Could you check a few things on this drawing? It's one solid part, dimensions in mm from its lowest x, y, z. A direction names the side the tool comes from. Give positions to 0.01 mm unless a question says otherwise; leave off trailing zeros. Order: outer loops, then holes, each group sorted by start corner. A loop starts at its lowest first (then second) coordinate and runs counter-clockwise, first axis right, second up.
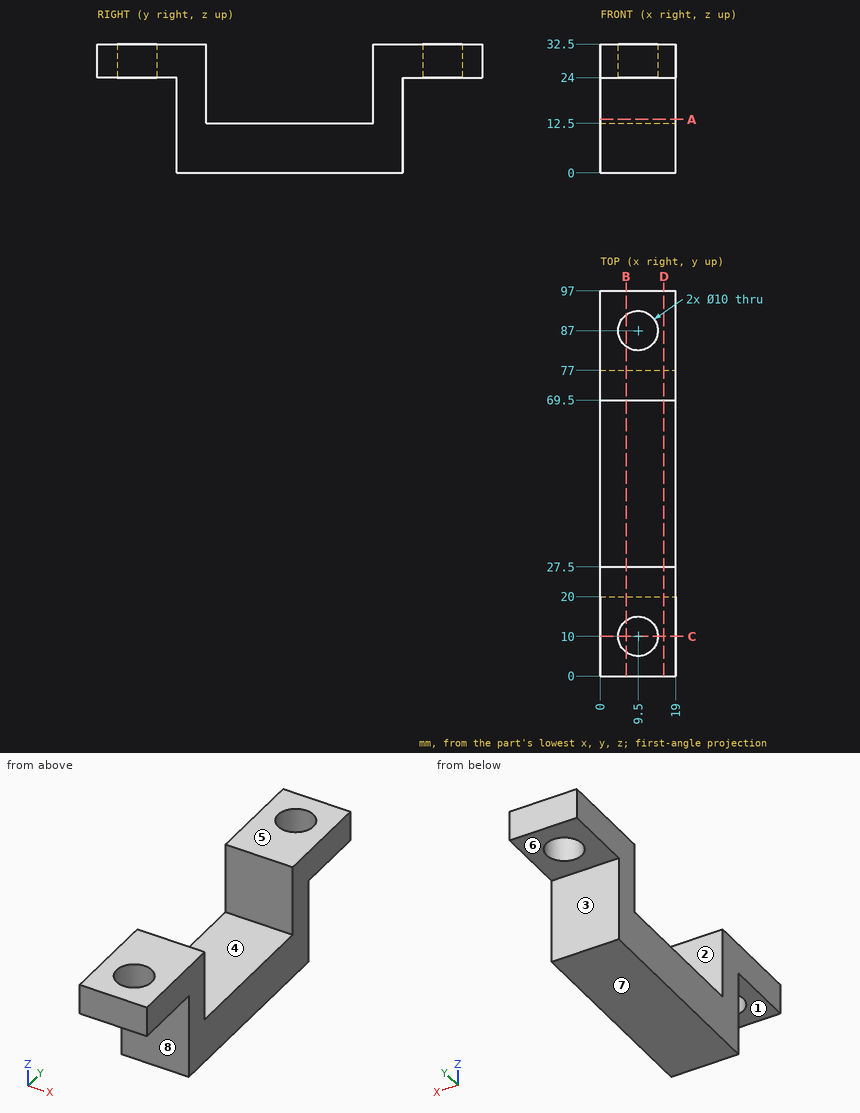
Q1. For the marked faces 4, 5, 6, 7 and 8, which set-ups out of +Z, -Z, +X, -X, +Y, -Y let a thin tool reach every point of the face, with its end or its side?
Filled sheet:
face 4: +Z, +X, -X
face 5: +Z, +X, -X, +Y, -Y
face 6: -Z, +X, -X, +Y
face 7: -Z, +X, -X, +Y, -Y
face 8: -Z, +X, -X, -Y
Q2. If we section it at A-A on z = 13.5: List the corners of the cut face in (x, y) for me.
Filled sheet:
outline: (0, 20) - (19, 20) - (19, 27.5) - (0, 27.5) - close; (0, 69.5) - (19, 69.5) - (19, 77) - (0, 77) - close
Q3. I'm going to push flat-ended pins straight in: P1, Ø9.5, axis at x = 5.5, z = 15, coming from the +Y side; P2, Ø9.5, axis at x = 13.5, y = 12, coming from the -Z side; P3, Ø9.5, axis at x = 12, z = 13, coming from the -Y side. Where does each tip first touch, or does it pass through?
Filled sheet:
P1: stops at y = 77
P2: stops at z = 24
P3: stops at y = 20
Q4. If we section it at C-C on y = 10: List the corners of the cut face in (x, z) for me.
Filled sheet:
outline: (0, 24) - (4.5, 24) - (4.5, 32.5) - (0, 32.5) - close; (14.5, 24) - (19, 24) - (19, 32.5) - (14.5, 32.5) - close
Q5. If we section it at D-D on x = 16: List the corners of the cut face in (y, z) for me.
Filled sheet:
outline: (0, 24) - (20, 24) - (20, 0) - (77, 0) - (77, 24) - (97, 24) - (97, 32.5) - (69.5, 32.5) - (69.5, 12.5) - (27.5, 12.5) - (27.5, 32.5) - (0, 32.5) - close
Q6. I need wall thicknesses on L1, parallel to Y at x = 9.5, z = 27.5; L2, parallel to Y at x = 13.5, z = 31; L3, parallel to Y at x = 2.75, z = 18. Which ranges of each line are inside material? Lowest first, please.
Filled sheet:
L1: y = 0 to 5, 15 to 27.5, 69.5 to 82, 92 to 97
L2: y = 0 to 7, 13 to 27.5, 69.5 to 84, 90 to 97
L3: y = 20 to 27.5, 69.5 to 77
Q7. If we section it at B-B on x = 6.5: List the corners of the cut face in (y, z) for me.
Filled sheet:
outline: (0, 24) - (6, 24) - (6, 32.5) - (0, 32.5) - close; (14, 24) - (20, 24) - (20, 0) - (77, 0) - (77, 24) - (83, 24) - (83, 32.5) - (69.5, 32.5) - (69.5, 12.5) - (27.5, 12.5) - (27.5, 32.5) - (14, 32.5) - close; (91, 24) - (97, 24) - (97, 32.5) - (91, 32.5) - close
Q8. Thinking about a two-plate mould opening in Y: for the marked faces 1, 2 and 3, which applies, released by +Y, released by -Y, zero draft, split by the parting line, or undercut?
Filled sheet:
face 1: zero draft
face 2: undercut
face 3: released by +Y
